Model file for the job. Use its own axes, mm. Give positions to 0.01 mm unless a question says otherwise; leave off trailing zeros. Order: outer loops, then holes, each group sorted by start corner. A loop starts at its lowest first (then second) coordinate and runs counter-clockwise, first axis right, second up. Notation, with made-up numbers: (-27, 73.25) - (-1, 73.25) arc R34 cw to (-1, 103.25) - close; hole circle Ø8 at (-14.5, -15.5). An arc over 180 degrees is marked (long way). Use CSV: the item, a comma, the result in double quotes. Start each with the question number.
(1) Band-saw the part on C-C, the plane z = 22. Give the cut face in (x, y).
(2) Band-saw the part on A-A, the plane x = 0. Give the cut face in (y, z).
(3) Probe L1, parallel to Y at x = 0, z = 16.5; L2, parallel to Y at x = -8.5, z = 13.5; L3, parallel to X at y = -31.5, z = 45. List the from-to ranges inside material, lowest first.
(4) Drop flat-ended pins along their axis: pin 1 Ø6 at (y, z) = (-10, 12) entering from -X; pin 2 Ø9 at (x, y) = (0, 0) entering from -Z; pin 3 Ø5 at (x, z) = (11, 34) entering from -Y. Give the stop position or say it passes through.
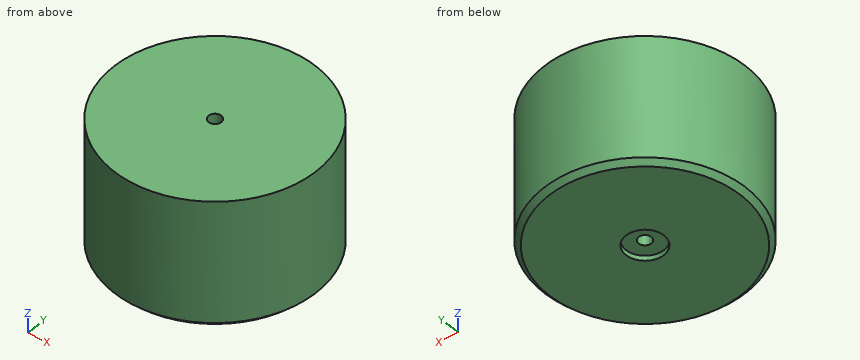
from build123d import *

# Parameters (mm, degrees)
F0_R     = 40
F1_DEPTH = 50
F2_R     = 2.5
F3_DEPTH = 50
F4_R     = 7.5
F5_DEPTH = 2
F6_SIZE  = 2


with BuildPart() as f1:
    # F0 (on Top) → F1 (new body)
    with BuildSketch(Plane.XY):
        Circle(F0_R)
    extrude(amount=F1_DEPTH)

    # F2 (on face) → F3 (cut)
    with BuildSketch(Plane.XY.offset(50)):
        Circle(F2_R)
    extrude(amount=-F3_DEPTH, mode=Mode.SUBTRACT)

    # F4 (on face) → F5 (cut)
    with BuildSketch(Plane(origin=(0, 0, 0), x_dir=(1, 0, 0), z_dir=(0, 0, -1))):
        Circle(F4_R)
    extrude(amount=-F5_DEPTH, mode=Mode.SUBTRACT)

    # F6
    f6_edges = [f1.edges().sort_by_distance(p)[0] for p in [
        (-40, 0, 0),
    ]]
    chamfer(f6_edges, length=F6_SIZE)


solid = f1.part
Answer block:
1,outline,"circle Ø80 at (0, 0); hole circle Ø5 at (0, 0)"
2,outline,"(-40, 2) - (-38, 0) - (-7.5, 0) - (-7.5, 2) - (-2.5, 2) - (-2.5, 50) - (-40, 50) - close; (2.5, 2) - (7.5, 2) - (7.5, 0) - (38, 0) - (40, 2) - (40, 50) - (2.5, 50) - close"
3,L1,"y = -40 to -2.5, 2.5 to 40"
3,L2,"y = -39.09 to 39.09"
3,L3,"x = -24.65 to 24.65"
4,pin 1,"stops at x = -39.38"
4,pin 2,"stops at z = 2"
4,pin 3,"stops at y = -39.09"
